from build123d import *

# Parameters (mm, degrees)
SKETCH_1_W          = 47.8
SKETCH_1_H          = 7.8
EXTRUDE_1_DEPTH     = 9.6
SKETCH_2_R          = 2.4
EXTRUDE_2_DEPTH     = 1.7
SKETCH_4_R          = 2.5
CUT_EXTRUDE_1_DEPTH = 1.8


with BuildPart() as part:
    # Эскиз1 → Бобышка-Вытянуть1 (new body)
    with BuildSketch(Plane.XY):
        Rectangle(SKETCH_1_W, SKETCH_1_H)
    extrude(amount=EXTRUDE_1_DEPTH)

    # Эскиз2 → Бобышка-Вытянуть2 (add)
    with BuildSketch(Plane(origin=(0, 0, 0), x_dir=(-1, 0, 0), z_dir=(0, 0, -1))):
        with Locations(Location((-20, 0, 0), (0, 0, 180))):
            Circle(SKETCH_2_R)
        with Locations(Location((-12, 0, 0), (0, 0, 180))):
            Circle(SKETCH_2_R)
        with Locations(Location((-4, 0, 0), (0, 0, 180))):
            Circle(SKETCH_2_R)
        with Locations(Location((4, 0, 0), (0, 0, 180))):
            Circle(SKETCH_2_R)
        with Locations(Location((12, 0, 0), (0, 0, 180))):
            Circle(SKETCH_2_R)
        with Locations(Location((20, 0, 0), (0, 0, 180))):
            Circle(SKETCH_2_R)
    extrude(amount=EXTRUDE_2_DEPTH)

    # Эскиз4 → Вырез-Вытянуть1 (cut)
    with BuildSketch(Plane.XY.offset(9.6)):
        with Locations((-20, 0)):
            Circle(SKETCH_4_R)
        with Locations((-12, 0)):
            Circle(SKETCH_4_R)
        with Locations((-4, 0)):
            Circle(SKETCH_4_R)
        with Locations((4, 0)):
            Circle(SKETCH_4_R)
        with Locations((12, 0)):
            Circle(SKETCH_4_R)
        with Locations((20, 0)):
            Circle(SKETCH_4_R)
    extrude(amount=-CUT_EXTRUDE_1_DEPTH, mode=Mode.SUBTRACT)


solid = part.part
The listing builds one solid part. Answer for the finished solid, in the listing's coordinates (mm). A direction names the side the tool comes from. Coordinates: 2 decimals unless noted, no trailing zeros. Order: outer loops, then holes, each group sorted by start corner. A loop starts at its lowest first (then second) coordinate and runs counter-clockwise, first axis right, second up.
Q1. A cutting plane is placed at C-C, the plane z = -1. Write down the section's boundary in (x, y), and give its area (3 significant figures).
Q2. Given P1, Ø4, axis at x = -12, y = 0, coming from the +Z side; P2, Ø1.5, axis at x = -1.5, y = 2, coming from the -Z side, each flat-ended and moving along its own axis, determine where each tip first touches the part or whether it passes through.
Q3. A cutting plane is placed at A-A, the plane z = 8.25. Write down the section's boundary in (x, y), and give its area (3 significant figures).
Q4. For a pull along Y with two mould halves and no side action, classify faces 1 (the face through (-1.615, 0.751, 8.713)), 2 (the face through (6.29, -0.72, -0.84)), 3 (the face through (0, 3.9, 5)), 4 (the face through (0, 0, 0)) as pulls with the +Y half, pulls with the -Y half, needs draft (parallel to the pull), parting line crosses it, or undercut.
Q5. Which of the six approach directions +Z, -Z, +X, -X, +Y, -Y give full straight-line access (tool end or side, diameter ignored) to faces 5 (the face through (-22.5, 0.1, 8.7)), 6 (the face through (-20, 0, -1.7)), 7 (the face through (-22.398, -0.106, -0.838))?
Q6. Consider line 1 (Y direction, x = -4, z = 8.75); line 2 (Z direction, x = -14, y = 2.75); line 3 (Y direction, x = 22, z = 8.5). Determine where each line is inside the solid, lowest interval first.
Q7. A cutting plane is placed at B-B, the plane x = 12. Write down the section's boundary in (y, z).
Answers follow:
1. outline: circle Ø4.8 at (-20, 0); circle Ø4.8 at (-12, 0); circle Ø4.8 at (-4, 0); circle Ø4.8 at (4, 0); circle Ø4.8 at (12, 0); circle Ø4.8 at (20, 0)
1. area: 109 mm2
2. P1: stops at z = 7.8
2. P2: stops at z = 0
3. outline: (-23.9, -3.9) - (23.9, -3.9) - (23.9, 3.9) - (-23.9, 3.9) - close; hole circle Ø5 at (-20, 0); hole circle Ø5 at (-12, 0); hole circle Ø5 at (-4, 0); hole circle Ø5 at (4, 0); hole circle Ø5 at (12, 0); hole circle Ø5 at (20, 0)
3. area: 255 mm2
4. face 1: undercut
4. face 2: parting line crosses it
4. face 3: pulls with the +Y half
4. face 4: needs draft
5. face 5: +Z
5. face 6: -Z, +X, -X, +Y, -Y
5. face 7: -Z
6. line 1: y = -3.9 to -2.5, 2.5 to 3.9
6. line 2: z = 0 to 9.6
6. line 3: y = -3.9 to -1.5, 1.5 to 3.9
7. outline: (-3.9, 0) - (-2.4, 0) - (-2.4, -1.7) - (2.4, -1.7) - (2.4, 0) - (3.9, 0) - (3.9, 9.6) - (2.5, 9.6) - (2.5, 7.8) - (-2.5, 7.8) - (-2.5, 9.6) - (-3.9, 9.6) - close
